Drawing for the job (mm, zero at the part's lowest x, y, z). A direction names the side the tool comes from. Round coordinates to 2 decimals unless told otherwise and drop trailing zeros. Loops run counter-clockwise (first coordinate to the right, second up) from the corner with the lowest first, then second, coordinate; pieces in that order, holes last. Notation, with made-up numbers: (44, 1.25) -> (78, 1.25) arc R22 ccw to (78, 20.25) -> close; hole circle Ø6 at (34.5, 18). An arc over 180 degrees is marked (long way). Put each result on its own line as item: value. Start each with the question number.
Item 1: Cut at B-B, the plane x = 86. List the corners of the cut face in (y, z) (1 decimal).
Item 2: Pull direction X, two halves, no side cores. Call the marked faces 1, 2 and 3: +X half, -X half, draft (parallel to the pull), parting line (faces both ways), or undercut.
Item 3: Flat gauge pins, fed straight in: pin 1 Ø10 at (x, z) = (61.5, 71.5) entering from -Y; pin 2 Ø14.5 at (x, y) = (135, 25.5) entering from -Z (3 decimals); pin 3 Ø22.5 at (x, y) = (20.5, 37.5) entering from +Z; pin 4 Ø12 at (x, y) = (55, 13) entering from +Z. Where does each tip first touch, or does it go through?
Item 4: Tool access for the marked faces 4 and 5: list every direction of +Z, -Z, +X, -X, +Y, -Y with a clear straight run to the whole face (end or side of a thin tool).
Item 5: Cut at A-A, the plane y = 69.5. List the corners of the cut face in (x, z) (1 decimal), plus the area to 3 significant figures.
Item 6: Cut at C-C, the plane z = 41. List the corners of the cut face in (x, y) (1 decimal).
Item 7: Drill centre lines: probe 1 along Z at (x, y) = (90, 19.5) (1 decimal); probe 2 along Z at (x, y) = (7, 11); probe 3 along X at (y, z) = (25, 24) (1 decimal). Where is each one in solid material? Low to high. Write a range as [from, to].
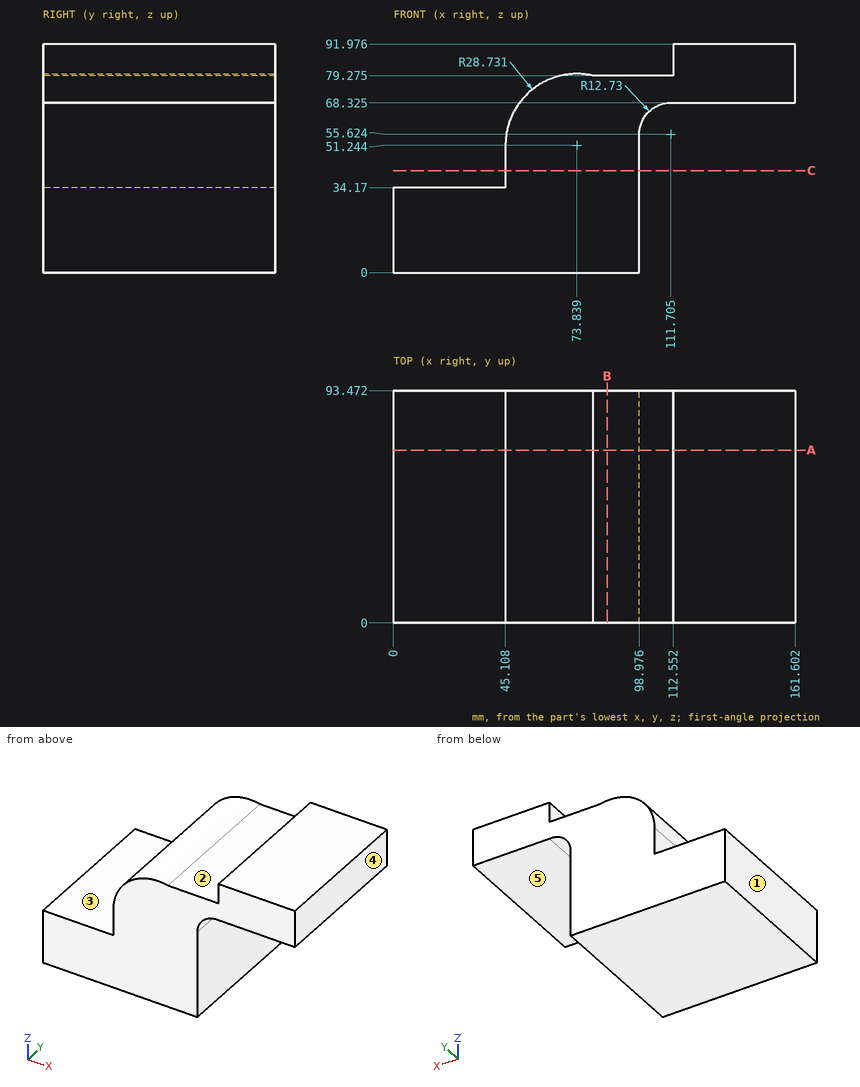
Reply:
1. outline: (0, 0) -> (93.5, 0) -> (93.5, 79.3) -> (0, 79.3) -> close
2. face 1: -X half
2. face 2: undercut
2. face 3: draft
3. pin 1: stops at y = 0
3. pin 2: stops at z = 68.325
3. pin 3: stops at z = 34.17
3. pin 4: stops at z = 76.95
4. face 4: +Z, -Z, +X, +Y, -Y
4. face 5: -Z, +X, +Y, -Y
5. outline: (0, 0) -> (99, 0) -> (99, 55.6) arc R12.7 cw to (112.6, 68.3) -> (161.6, 68.3) -> (161.6, 92) -> (112.6, 92) -> (112.6, 79.3) -> (80.1, 79.3) arc R28.7 ccw to (45.1, 51.2) -> (45.1, 34.2) -> (0, 34.2) -> close
5. area: 7,000 mm^2
6. outline: (45.1, 0) -> (99, 0) -> (99, 93.5) -> (45.1, 93.5) -> close
7. probe 1: z = [0, 79.3]
7. probe 2: z = [0, 34.17]
7. probe 3: x = [0, 99]
